from build123d import *


with BuildPart() as f1:
    # F0 (on Right) → F1 (revolve)
    with BuildSketch(Plane.YZ):
        with BuildLine():
            Line((63.5, 3.5), (63.5, 0))
            Line((63.5, 0), (73.5, 0))
            ThreePointArc((73.5, 0), (77.3359133031, 1.5134897068), (80.9495899372, 3.5))
            Line((80.9495899372, 3.5), (63.5, 3.5))
        make_face()
        with BuildLine():
            ThreePointArc((80.9495899372, 3.5), (77.3359133031, 1.5134897068), (73.5, 0))
            Line((73.5, 0), (81.9394091831, 0))
            ThreePointArc((81.9394091831, 0), (99.4102229196, 33.9875285278), (76.5, 64.5735239147))
            Line((76.5, 64.5735239147), (76.5, 60.7901444396))
            ThreePointArc((76.5, 60.7901444396), (90.7182725546, 48.7908944847), (96.0374015748, 30.9625984252))
            ThreePointArc((96.0374015748, 30.9625984252), (92.017072223, 15.2954642562), (80.9495899372, 3.5))
        make_face()
    revolve(axis=Axis((0, 63.5, 33.5), (0, 0, -1)))

    # F3 (on line) → F4 (revolve, cut)
    with BuildSketch(Plane(origin=(0, 63.5, 0), x_dir=(-1, 0, 0), z_dir=(0, 1, 0))):
        Polygon((-27.3694280028, 58.332026428), (-21.2339044516, 52.1965028768), (-19.112584108, 54.3178232204), (-25.2481076593, 60.4533467716), align=None)
    revolve(axis=Axis((15.2781799182, 63.5, 46.2407783434), (0.7071067812, 0, 0.7071067812)), mode=Mode.SUBTRACT)


solid = f1.part
Design review of the part built by this model. Coordinates are the model's own, in mm. Round coordinates to 2 decimals unless told otherwise and drop trailing zeros. Loops run counter-clockwise (first coordinate to the right, second up) from the corner with the lowest first, then second, coordinate; pieces in that order, holes last. Notation, with made-up numbers: (34.5, -38.75) - (56.5, -38.75) arc R16 cw to (56.5, -26.75) - close; hole circle Ø5 at (54.25, 66.25). An arc over 180 degrees is marked (long way). One line per question, with ' | ' between items.
1. We need section D-D, the plane x = 11.5. State the section outline as (y, z) points.
Results are:
outline: (49.09, 0) - (77.91, 0) arc R34.15 ccw to (69.56, 64.57) - (69.56, 60.79) arc R30.44 cw to (76.62, 3.5) - (50.38, 3.5) arc R30.44 cw to (57.44, 60.79) - (57.44, 64.57) arc R34.15 ccw to start
2. We need section A-A, the plane y = 63.5. State the section outline as (x, z) points.
Results are:
outline: (-18.44, 0) - (18.44, 0) arc R36.04 ccw to (27.52, 54.24) - (25.03, 51.75) arc R32.54 cw to (17.45, 3.5) - (-17.45, 3.5) arc R32.54 cw to (-13, 60.79) - (-13, 64.57) arc R36.04 ccw to start; (13, 60.79) arc R32.54 cw to (20.79, 55.99) - (23.27, 58.48) arc R36.04 ccw to (13, 64.57) - close
3. For L1, parallel to X at y = 57, z = 23.5; L2, parallel to Y at x = -22.5, z = 25 (3 decimals); L3, parallel to Z at x = 17.5, y = 49.5, list the stretches that pass through material, from the lowest coordinate up. Write a range as [from, to].
Results are:
L1: x = [-34.65, -31], [31, 34.65] | L2: y = [35.988, 40.765], [86.235, 91.012] | L3: z = [2.74, 7.37], [54.55, 59.18]
4. We need section C-C, the plane y = 85.5. State the section outline as (x, z) points.
Results are:
outline: circle Ø57.09 at (0, 30.96); hole circle Ø47.95 at (0, 30.96)
5. Clearance check with flat-ended pins moving along their axes: P1, Ø17.5, axis at x = 4.5, y = 64.5, coming from the +Z side; P2, Ø10, axis at x = -10, z = 40, coming from the -Y side; P3, Ø5, axis at x = 24.5, z = 9, coming from the +Y side; P4, Ø5, axis at x = -25.5, z = 10.5, coming from the -Y side. State where each tip first meets the part, or that it passes through.
Results are:
P1: stops at z = 64.57 | P2: stops at y = 28.47 | P3: stops at y = 82.85 | P4: stops at y = 43.83
6. Draft analysis for pull direction Y (two halves, no side actions). For faces 1 (the face through (0.572, 50.513, 62.655)), 2 (the face through (0, 64, 0)), state which applies: released by +Y, released by -Y, zero draft, split by the parting line, or undercut.
Results are:
face 1: undercut | face 2: zero draft
7. We need section B-B, the plane x = 0. State the section outline as (y, z) points.
Results are:
outline: (45.06, 0) - (81.94, 0) arc R36.04 ccw to (76.5, 64.57) - (76.5, 60.79) arc R32.54 cw to (80.95, 3.5) - (46.05, 3.5) arc R32.54 cw to (50.5, 60.79) - (50.5, 64.57) arc R36.04 ccw to start
